Part print with two shaded views. Sizes in mm from the minimum x, y, z corner. A direction names the side the tool comes from. Coordinates: 2 decimals unless noted, no trailing zeros. Write each loop counter-clockwise with the first axis right and the second up, starting at its lowest first coordinate (ties: lowest second). Pieces come first, ordered by that corner, then holes. Notation, with made-up numbers: M -35,63 L 12,63 A34 ccw 12,98 Z; hole C -12,78 d6. An arc over 180 degrees is marked long. Answer in a Markdown table with one row per item. Add a question column.
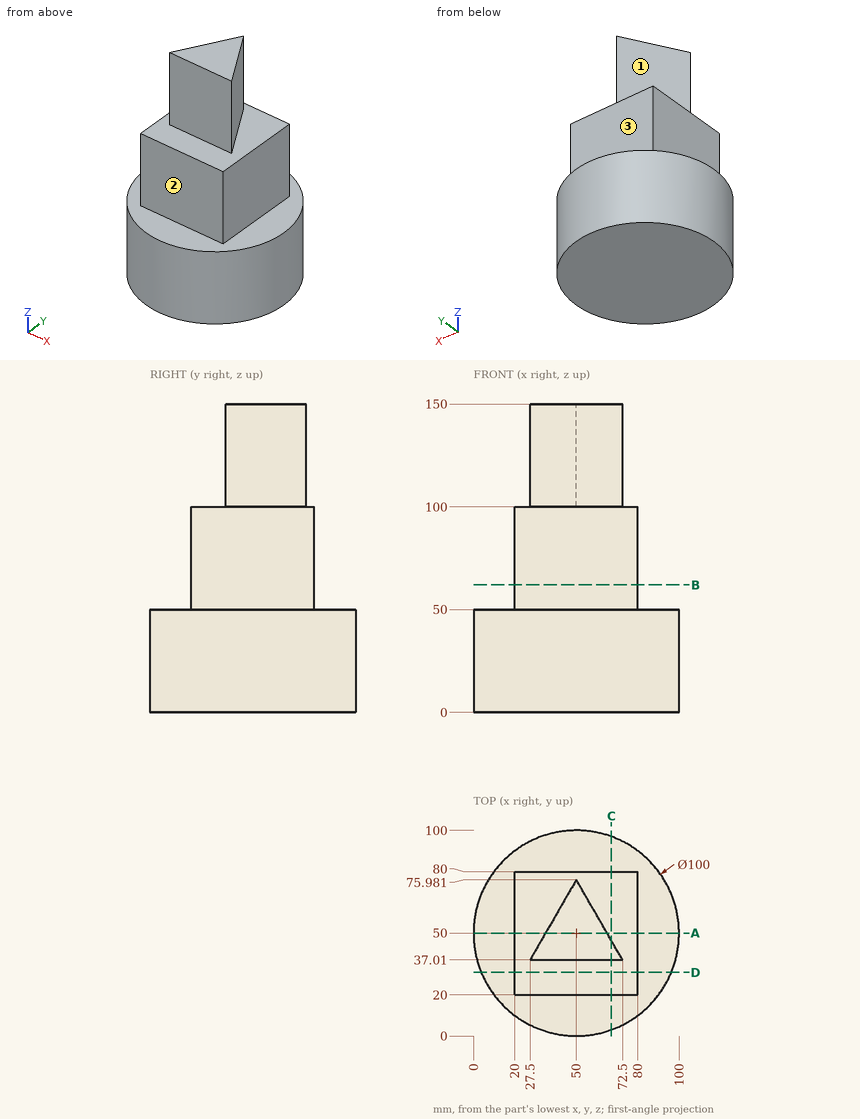
1) Slice it at A-A (y = 50). Give the cut face in (x, z), then the cut area to 3 significant figures.
2) Drill centre lines: probe 1 along Z at (x, y) = (68, 23); probe 2 along Z at (x, y) = (56.5, 83.5); probe 3 along Y at (x, z) = (49, 17.5). Where is each one in solid material? Low to high.
3) Slice it at C-C (x = 67). Give the cut face in (y, z), then the cut area to 3 significant figures.
4) Slice it at B-B (z = 62). Give the cut face in (x, y).
5) Which spindle directions (+Z, -Z, +X, -X, +Y, -Y) get a long thin tool onto all of the face, cutting with end or side? Do the marked faces 1, 2 and 3. Say none if no direction does.
6) Slice it at D-D (y = 31). Give the cut face in (x, z), then the cut area to 4 significant figures.
7) Flat gauge pins, fed straight in: pin 1 Ø15 at (x, z) = (36.5, 62.5) entering from -Y; pin 2 Ø15 at (y, z) = (47, 70) entering from -X; pin 3 Ø6 at (x, y) = (13.5, 40.5) entering from +Z. Where does each tip first touch, or does it go through?
Ans:
| question | item | result |
|---|---|---|
| 1 | outline | M 0,0 L 100,0 L 100,50 L 80,50 L 80,100 L 65,100 L 65,150 L 35,150 L 35,100 L 20,100 L 20,50 L 0,50 Z |
| 1 | area | 9,500 mm2 |
| 2 | probe 1 | z = 0 to 100 |
| 2 | probe 2 | z = 0 to 50 |
| 2 | probe 3 | y = 0.01 to 99.99 |
| 3 | outline | M 2.98,0 L 97.02,0 L 97.02,50 L 80,50 L 80,100 L 46.54,100 L 46.54,150 L 37.01,150 L 37.01,100 L 20,100 L 20,50 L 2.98,50 Z |
| 3 | area | 8,180 mm2 |
| 4 | outline | M 20,20 L 80,20 L 80,80 L 20,80 Z |
| 5 | face 1 | +Z, -X, +Y |
| 5 | face 2 | +Z, +X, -X, -Y |
| 5 | face 3 | +Z, +X, -X, +Y |
| 6 | outline | M 3.75,0 L 96.25,0 L 96.25,50 L 80,50 L 80,100 L 20,100 L 20,50 L 3.75,50 Z |
| 6 | area | 7,625 mm2 |
| 7 | pin 1 | stops at y = 20 |
| 7 | pin 2 | stops at x = 20 |
| 7 | pin 3 | stops at z = 50 |
